from build123d import *

# Parameters (mm, degrees)
SKETCH_W      = 17
SKETCH_H      = 34
SKETCH_R      = 1.5
SKETCH_R_2    = 1
PAD_DEPTH     = 1.5
SKETCH001_W   = 17
SKETCH001_H   = 1.5
PAD001_DEPTH  = 30
SKETCH002_R   = 1.5
SKETCH002_R_2 = 1
POCKET_DEPTH  = 34.001


with BuildPart() as part:
    # Sketch → Pad (new body)
    with BuildSketch(Plane.XY):
        with Locations((8.5, 17)):
            Rectangle(SKETCH_W, SKETCH_H)
        with Locations((8.5, 17)):
            Circle(SKETCH_R, mode=Mode.SUBTRACT)
        with Locations((8.5, 10.5)):
            Circle(SKETCH_R_2, mode=Mode.SUBTRACT)
        with Locations((8.5, 23.5)):
            Circle(SKETCH_R_2, mode=Mode.SUBTRACT)
    extrude(amount=PAD_DEPTH)

    # Sketch001 → Pad001 (new body)
    with BuildSketch(Plane.XY):
        with Locations((8.5, 0.75)):
            Rectangle(SKETCH001_W, SKETCH001_H)
    extrude(amount=PAD001_DEPTH)

    # Sketch002 → Pocket (cut, through all)
    with BuildSketch(Plane.XZ):
        with Locations((8.5, 16.5)):
            Circle(SKETCH002_R)
        with Locations((8.5, 10.5)):
            Circle(SKETCH002_R_2)
        with Locations((8.5, 22.5)):
            Circle(SKETCH002_R_2)
    extrude(amount=-POCKET_DEPTH, mode=Mode.SUBTRACT)


solid = part.part
Verification items for the finished model (mm, model axes). A direction names the side the tool comes from. Coordinates: 2 decimals unless noted, no trailing zeros. Loops run counter-clockwise (first coordinate to the right, second up) from the corner with the lowest first, then second, coordinate; pieces in that order, holes last. Notation, with made-up numbers: (33.5, 39.25) -> (70.5, 39.25) arc R22 ccw to (70.5, 76.25) -> close; hole circle Ø1 at (68.25, -8). An arc over 180 degrees is marked (long way). Answer as a JSON object with one key per item and string values. Group by question number.
Item 1: Tool access check on faces 1 (the flat face through (6, 18, 1.5)), 2 (the cylindrical face through (7.39, 0.74, 17.51)). Record the directions out of +Z, -Z, +X, -X, +Y, -Y that give a thin tool (end or side, any length) a straight path to the whole face; none if there is none.
Item 2: Scan lines: probe 1 along Y at (x, z) = (8.5, 0.8); probe 2 along Z at (x, y) = (8.5, 0.45); probe 3 along Y at (x, z) = (5.5, 11). Record each from-to range of solid material in increasing order.
Item 3: Mould release check, pull along Y, two halves, no side actions. Record for faces 3 (the cylindrical face through (7.39, 18.01, 0.74)), 4 (the flat face through (8, 1, 30)), 5 (the flat face through (6, 1.5, 16)): +Y half, -Y half, draft (parallel to the pull), parting line (faces both ways), or undercut.
Item 4: Depth check by flat-ended pin: pin 1 (5 mm diameter, centred on x = 8, y = 10, fed in from +Z). Enter the tip coordinate at first touch or a pass-through.
Item 5: Sectioned sample at C-C on x = 8.5. State how many separate pieces and enclosed holes the cut face has, plus the area to 4 significant figures.
Item 6: Sectioned sample at A-A on y = 17. Record the boundary of the cut face in (x, z).
Item 7: Sectioned sample at D-D on y = 4. Record the boundary of the cut face in (x, z), plus the area to 3 significant figures.
Evaluation:
{
 "1": {"face 1": "+Z, +X, -X, +Y", "face 2": "+Y, -Y"},
 "2": {"probe 1": "y = 0 to 9.5, 11.5 to 15.5, 18.5 to 22.5, 24.5 to 34", "probe 2": "z = 0 to 9.5, 11.5 to 15, 18 to 21.5, 23.5 to 30", "probe 3": "y = 0 to 1.5"},
 "3": {"face 3": "undercut", "face 4": "draft", "face 5": "+Y half"},
 "4": {"pin 1": "stops at z = 1.5"},
 "5": {"separate pieces": "7", "enclosed holes": "0", "area": "72.75 mm²"},
 "6": {"outline": "(0, 0) -> (7, 0) -> (7, 1.5) -> (0, 1.5) -> close; (10, 0) -> (17, 0) -> (17, 1.5) -> (10, 1.5) -> close"},
 "7": {"outline": "(0, 0) -> (17, 0) -> (17, 1.5) -> (0, 1.5) -> close", "area": "25.5 mm²"}
}
